```python
from build123d import *

# Parameters (mm, degrees)
SKETCH001_R       = 0.45
PAD001_DEPTH      = 10
PAD001_DEPTH_BACK = 3.5
SKETCH_R          = 6
PAD_DEPTH         = 20
FILLET_R          = 0.5


with BuildPart() as pad001:
    # Sketch001 → Pad001 (new body, two sides)
    with BuildSketch(Plane.XY.offset(0.5)) as pad001_sk:
        Circle(SKETCH001_R)
        with Locations((5, 0)):
            Circle(SKETCH001_R)
    extrude(amount=PAD001_DEPTH)
    extrude(pad001_sk.sketch, amount=-PAD001_DEPTH_BACK)


with BuildPart() as obj1:
    # Sketch → Pad (new body)
    with BuildSketch(Plane.XY.offset(0.1)):
        with Locations((2.5, 0)):
            Circle(SKETCH_R)
    extrude(amount=PAD_DEPTH)

    # Fillet
    fillet_edges = [obj1.edges().sort_by_distance(p)[0] for p in [
        (-3.5, 0, 0.1),
        (-3.5, 0, 20.1),
    ]]
    fillet(fillet_edges, radius=FILLET_R)

    # obj1: union Pad001
    add(pad001.part)


solid = obj1.part
```
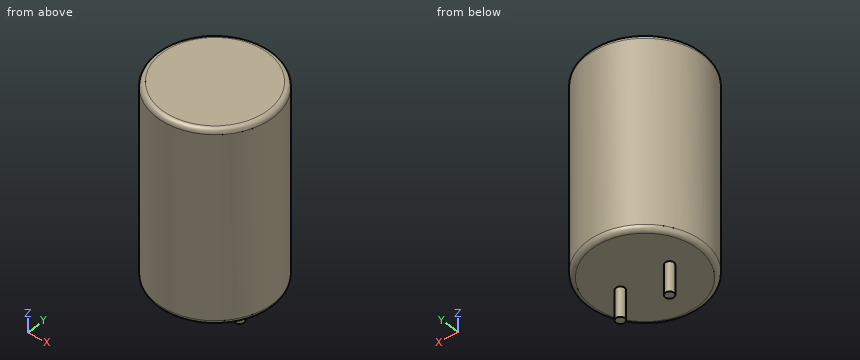
Geometry: final body of the model. Coordinates: model frame, mm. Coordinates: 2 decimals unless noted, no trailing zeros. Loops run counter-clockwise (first coordinate to the right, second up) from the corner with the lowest first, then second, coordinate; pieces in that order, holes last. Notation, with made-up numbers: (39, 83.5) -> (76, 83.5) arc R17 cw to (76, 113.5) -> close; hole circle Ø2 at (72.25, 53). An arc over 180 degrees is marked (long way). Use a Markdown table: item, result. Add a question column.
(1) Section query C-C, the plane z = 8. Return loops of the section in (x, y), plus the area to 3 significant figures.
(2) Section query A-A, the plane x = 2.5. Return loops of the section in (y, z).
(3) Pin query (flat end, axial travel): pin 1 Ø2 at (x, z) = (1, 7) entering from +Y; pin 2 Ø1.5 at (x, y) = (1.5, -4) entering from -Z; pin 3 Ø3 at (y, z) = (-4.5, 14.5) entering from +X. Return the tip coordinate at first contact, or that it passes through.
(4) Section query B-B, the plane y = 0. Return loops of the section in (x, z), plus the area to 3 significant figures.
(5) Line query: line 1 along Z through (x, y) = (-1, 3.75); line 2 along X through (y, z) = (1.5, 2.25); line 3 along X through (y, z) = (-4.25, 15.5). Output: solid intervals per line, ascending.
Answer:
| question | item | result |
|---|---|---|
| 1 | outline | circle Ø12 at (2.5, 0) |
| 1 | area | 113 mm^2 |
| 2 | outline | (-6, 0.6) arc R0.5 ccw to (-5.5, 0.1) -> (5.5, 0.1) arc R0.5 ccw to (6, 0.6) -> (6, 19.6) arc R0.5 ccw to (5.5, 20.1) -> (-5.5, 20.1) arc R0.5 ccw to (-6, 19.6) -> close |
| 3 | pin 1 | stops at y = 5.98 |
| 3 | pin 2 | stops at z = 0.1 |
| 3 | pin 3 | stops at x = 7.7 |
| 4 | outline | (-3.5, 0.6) arc R0.5 ccw to (-3, 0.1) -> (-0.45, 0.1) -> (-0.45, -3) -> (0.45, -3) -> (0.45, 0.1) -> (4.55, 0.1) -> (4.55, -3) -> (5.45, -3) -> (5.45, 0.1) -> (8, 0.1) arc R0.5 ccw to (8.5, 0.6) -> (8.5, 19.6) arc R0.5 ccw to (8, 20.1) -> (-3, 20.1) arc R0.5 ccw to (-3.5, 19.6) -> close |
| 4 | area | 245 mm^2 |
| 5 | line 1 | z = 0.1 to 20.1 |
| 5 | line 2 | x = -3.31 to 8.31 |
| 5 | line 3 | x = -1.74 to 6.74 |
